```python
from build123d import *

# Parameters (mm, degrees)
VYSUNOUT1_DEPTH = 7
SKICA5_R        = 5
VYSUNOUT4_DEPTH = 28
ZKOSIT1_SIZE    = 0.7
SKICA3_R        = 5.3
VYSUNOUT2_DEPTH = 1
SKICA4_R        = 5.5
VYSUNOUT3_DEPTH = 9.12


with BuildPart() as part:
    # Skica1 → Vysunout1 (new body)
    with BuildSketch(Plane.XY):
        Polygon((8, -4.618802154), (8, 4.618802154), (0, 9.237604307), (-8, 4.618802154), (-8, -4.618802154), (0, -9.237604307), align=None)
    extrude(amount=VYSUNOUT1_DEPTH)

    # Skica2 → Odebrat otočením1 (revolve, cut)
    with BuildSketch(Plane(origin=(0, 0, 0), x_dir=(1, 0, 0), z_dir=(0, 1, 0))):
        Polygon((8, 0), (20.124355653, 0), (20.124355653, -7), align=None)
    revolve(axis=Axis((0, 0, 0), (0, 0, 1)), mode=Mode.SUBTRACT)

    # Skica5 → Vysunout4 (add)
    with BuildSketch(Plane.XY.offset(7)):
        Circle(SKICA5_R)
    extrude(amount=VYSUNOUT4_DEPTH)

    # Zkosit1
    zkosit1_edges = [part.edges().sort_by_distance(p)[0] for p in [
        (-5, 0, 35),
    ]]
    chamfer(zkosit1_edges, length=ZKOSIT1_SIZE)

    # Skica3 → Vysunout2 (add)
    with BuildSketch(Plane.XY.offset(7)):
        Circle(SKICA3_R)
    extrude(amount=VYSUNOUT2_DEPTH)

    # Skica4 → Vysunout3 (add)
    with BuildSketch(Plane.XY.offset(8)):
        Circle(SKICA4_R)
    extrude(amount=VYSUNOUT3_DEPTH)

    # Skica6 → Odebrat otočením2 (revolve, cut)
    with BuildSketch(Plane(origin=(0, 0, 0), x_dir=(1, 0, 0), z_dir=(0, 1, 0)), mode=Mode.PRIVATE) as odebrat_oto_en_m2_sk:
        Polygon((-5.5, -17.12), (-5.5, -16.253974596), (-5, -17.12), align=None)
    revolve(odebrat_oto_en_m2_sk.sketch.rotate(Axis((0, 0, 17.12), (0, 0, -1)), 180), axis=Axis((0, 0, 17.12), (0, 0, -1)), mode=Mode.SUBTRACT)

    # Skica7 → Otočit kolem osy1 (revolve)
    with BuildSketch(Plane(origin=(0, 0, 0), x_dir=(1, 0, 0), z_dir=(0, 1, 0))):
        with BuildLine():
            ThreePointArc((5.3, -7.4), (5.321093687, -7.195690356), (5.383484861, -7))
            Line((5.383484861, -7), (5.3, -7))
            Line((5.3, -7), (5.3, -7.4))
        make_face()
        with BuildLine():
            ThreePointArc((5.5, -8), (5.351316702, -7.716227766), (5.3, -7.4))
            Line((5.3, -7.4), (5.3, -8))
            Line((5.3, -8), (5.5, -8))
        make_face()
    revolve(axis=Axis((0, 0, 16.253974596), (0, 0, -1)))


solid = part.part
```
The model under review builds one solid part; all positions refer to its coordinate system, in mm. A direction names the side the tool comes from. Give positions to 0.01 mm unless a question says otherwise; leave off trailing zeros. Write each loop counter-clockwise with the first axis right and the second up, starting at its lowest first coordinate (ties: lowest second). Pieces come first, ordered by that corner, then holes. Notation, with made-up numbers: M 68.25,21 L 113.25,21 A19 cw 113.25,57 Z; hole C 82.25,87.25 d2. An arc over 180 degrees is marked long. Write each question's results on one line, items separated by ' | '. Start each with the question number.
1. Mouldability with a two-part tool opening along Y and no side actions: class faces 3 (the flat face through (-4.056, -6.896, 3.451)), 4 (the flat face through (8, 0, 3)), 5 (the cylindrical face through (-1.19, -5.37, 12.07)) as released by +Y, released by -Y, zero draft, split by the parting line, or undercut.
2. Insertion check: pin 1 Ø1 at (x, z) = (-1.5, 31.5) entering from -Y; pin 2 Ø4 at (x, z) = (-1, 21) entering from -Y; pin 3 Ø6 at (x, y) = (6, -1) entering from +Z; pin 4 Ø8 at (y, z) = (-6, 14.5) entering from -X. Each pin has a flat end and moves straight along its axis. Give the tip position at first contact, or say it passes through.
3. We need section A-A (z = 19). Write out the cut boundary in (x, y), and give its area (3 significant figures).
4. For probe 1 along X at (y, z) = (3, 26); probe 2 along X at (y, z) = (6.75, 6), list the stretches that pass through material, from the lowest coordinate up. Write a range as [from, to].
5. For faces 1 (the conical face through (0.02, 8.295, 0.17)), 2 (the cylindrical face through (-1.08, -4.88, 25.59)), list the 3-axis set-ups (+Z, -Z, +X, -X, +Y, -Y) from which the entire face can be reached by the end or side of a thin tool; tool diameter is ignored.
Results found:
1) face 3: released by -Y | face 4: zero draft | face 5: split by the parting line
2) pin 1: stops at y = -4.9 | pin 2: stops at y = -5 | pin 3: stops at z = 35 | pin 4: stops at x = -5.12
3) outline: C 0,0 d10 | area: 78.5 mm^2
4) probe 1: x = [-4, 4] | probe 2: x = [-4.31, 4.31]
5) face 1: -Z, +Y | face 2: +Z
